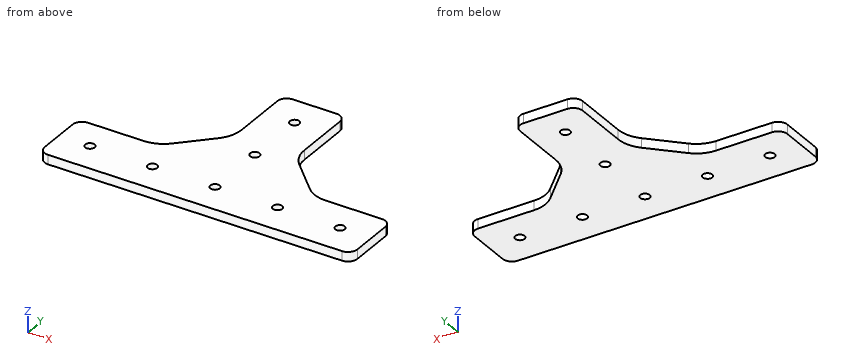
from build123d import *

# Parameters (mm, degrees)
SKETCH_1_W          = 20
SKETCH_1_H          = 60
EXTRUDE_1_DEPTH     = 3
SKETCH_2_W          = 60
SKETCH_2_H          = 20
EXTRUDE_2_DEPTH     = 3
SKETCH_3_W          = 60
SKETCH_3_H          = 20
EXTRUDE_3_DEPTH     = 3
SKETCH_4_R          = 1.5
CUT_EXTRUDE_1_DEPTH = 3
FILLET_2_R          = 3
CHAMFER_1_SIZE      = 15
FILLET_3_R          = 10


with BuildPart() as part:
    # 草图1 → 凸台-拉伸1 (new body)
    with BuildSketch(Plane.XY):
        with Locations((10, 30)):
            Rectangle(SKETCH_1_W, SKETCH_1_H)
    extrude(amount=EXTRUDE_1_DEPTH)

    # 草图2 → 凸台-拉伸2 (add)
    with BuildSketch(Plane.XY.offset(3)):
        with Locations((30, 10)):
            Rectangle(SKETCH_2_W, SKETCH_2_H)
    extrude(amount=-EXTRUDE_2_DEPTH)

    # 草图3 → 凸台-拉伸3 (add)
    with BuildSketch(Plane.XY.offset(3)):
        with Locations((-10, 10)):
            Rectangle(SKETCH_3_W, SKETCH_3_H)
    extrude(amount=-EXTRUDE_3_DEPTH)

    # 草图4 → 切除-拉伸1 (cut)
    with BuildSketch(Plane.XY.offset(3)):
        with Locations((10, 10)):
            Circle(SKETCH_4_R)
        with Locations((10, 30)):
            Circle(SKETCH_4_R)
        with Locations((10, 50)):
            Circle(SKETCH_4_R)
        with Locations((-30, 10)):
            Circle(SKETCH_4_R)
        with Locations((-10, 10)):
            Circle(SKETCH_4_R)
        with Locations((30, 10)):
            Circle(SKETCH_4_R)
        with Locations((50, 10)):
            Circle(SKETCH_4_R)
    extrude(amount=-CUT_EXTRUDE_1_DEPTH, mode=Mode.SUBTRACT)

    # 圆角2
    fillet_2_edges = [part.edges().sort_by_distance(p)[0] for p in [
        (60, 0, 1.5),
        (60, 20, 1.5),
        (-40, 20, 1.5),
        (-40, 0, 1.5),
        (0, 60, 1.5),
        (20, 60, 1.5),
    ]]
    fillet(fillet_2_edges, radius=FILLET_2_R)

    # 倒角1
    chamfer_1_edges = [part.edges().sort_by_distance(p)[0] for p in [
        (20, 20, 1.5),
        (0, 20, 1.5),
    ]]
    chamfer(chamfer_1_edges, length=CHAMFER_1_SIZE)

    # 圆角3
    fillet_3_edges = [part.edges().sort_by_distance(p)[0] for p in [
        (20, 35, 1.5),
        (35, 20, 1.5),
        (0, 35, 1.5),
        (-15, 20, 1.5),
    ]]
    fillet(fillet_3_edges, radius=FILLET_3_R)


solid = part.part
Work out the finished part from the listing and answer in its coordinate system (mm). Give positions to 0.01 mm unless a question says otherwise; leave off trailing zeros. Order: outer loops, then holes, each group sorted by start corner. A loop starts at its lowest first (then second) coordinate and runs counter-clockwise, first axis right, second up. Notation, with made-up numbers: (47.5, -26) -> (51.5, -26) arc R15 ccw to (51.5, -19) -> close; hole circle Ø3 at (31.25, 78). An arc over 180 degrees is marked (long way). Answer as a JSON object with one key per item and string values. Group by question number.
1. Section A-A on y = 10 is taken. Determine the outline of the cut face in (x, z).
2. Flat-ended cylindrical pins translate along their axes: pin 1 Ø1.5 at (y, z) = (49.5, 2) entering from -X; pin 2 Ø1.5 at (x, z) = (44, 1.5) entering from +Y; pin 3 Ø1.5 at (x, z) = (1.5, 1.5) entering from +Y. Find the tip coordinate at first contact, or state that the pin passes through.
3. Section D-D on z = 2.5 is taken. Determine the outline of the cut face in (x, y), plus the area to 3 significant figures.
4. Consider line 1 along Y through (x, z) = (10, 2.3); line 2 along X through (y, z) = (53.5, 1.1). Determine where each line is inside the solid, lowest interval first. Write a range as [from, to].
5. Section C-C on y = 30 is taken. Determine the outline of the cut face in (x, z).
6. Section B-B on x = 30 is taken. Determine the outline of the cut face in (y, z).
Result sheet:
{
 "1": {"outline": "(-40, 0) -> (-31.5, 0) -> (-31.5, 3) -> (-40, 3) -> close; (-28.5, 0) -> (-11.5, 0) -> (-11.5, 3) -> (-28.5, 3) -> close; (-8.5, 0) -> (8.5, 0) -> (8.5, 3) -> (-8.5, 3) -> close; (11.5, 0) -> (28.5, 0) -> (28.5, 3) -> (11.5, 3) -> close; (31.5, 0) -> (48.5, 0) -> (48.5, 3) -> (31.5, 3) -> close; (51.5, 0) -> (60, 0) -> (60, 3) -> (51.5, 3) -> close"},
 "2": {"pin 1": "stops at x = 0", "pin 2": "stops at y = 20", "pin 3": "stops at y = 59.9"},
 "3": {"outline": "(-40, 3) arc R3 ccw to (-37, 0) -> (57, 0) arc R3 ccw to (60, 3) -> (60, 17) arc R3 ccw to (57, 20) -> (39.14, 20) arc R10 cw to (32.07, 22.93) -> (22.93, 32.07) arc R10 cw to (20, 39.14) -> (20, 57) arc R3 ccw to (17, 60) -> (3, 60) arc R3 ccw to (0, 57) -> (0, 39.14) arc R10 cw to (-2.93, 32.07) -> (-12.07, 22.93) arc R10 cw to (-19.14, 20) -> (-37, 20) arc R3 ccw to (-40, 17) -> close; hole circle Ø3 at (-30, 10); hole circle Ø3 at (-10, 10); hole circle Ø3 at (10, 10); hole circle Ø3 at (10, 30); hole circle Ø3 at (10, 50); hole circle Ø3 at (30, 10); hole circle Ø3 at (50, 10)", "area": "2,970 mm^2"},
 "4": {"line 1": "y = [0, 8.5], [11.5, 28.5], [31.5, 48.5], [51.5, 60]", "line 2": "x = [0, 20]"},
 "5": {"outline": "(-5, 0) -> (8.5, 0) -> (8.5, 3) -> (-5, 3) -> close; (11.5, 0) -> (25, 0) -> (25, 3) -> (11.5, 3) -> close"},
 "6": {"outline": "(0, 0) -> (8.5, 0) -> (8.5, 3) -> (0, 3) -> close; (11.5, 0) -> (25, 0) -> (25, 3) -> (11.5, 3) -> close"}
}
